from build123d import *

# Parameters (mm, degrees)
SKETCH_1_W               = 115
SKETCH_1_H               = 30
EXTRUDE_1_DEPTH          = 29
SHELL_1_T                = -2
SKETCH_4_W               = 55
SKETCH_4_H               = 63
EXTRUDE_2_DEPTH          = 2
SKETCH_7_W               = 28
SKETCH_7_H               = 49
CUT_EXTRUDE_2_DEPTH      = 28
EXTRUDE_6_DEPTH          = 29
EXTRUDE_8_DEPTH          = 2
EXTRUDE_9_DEPTH          = 115
FILLET_1_R               = 1
SKETCH_8_R               = 1.2
CUT_EXTRUDE_5_DEPTH      = 10
SKETCH_15_W              = 113
SKETCH_15_H              = 39.979543783
CUT_EXTRUDE_6_DEPTH      = 33
CUT_EXTRUDE_7_REACH      = 152.193
SKETCH_16_W              = 16.4
SKETCH_16_H              = 9.3
SKETCH_17_W              = 40.5
SKETCH_17_H              = 2
EXTRUDE_10_DEPTH         = 113
CUT_EXTRUDE_8_DEPTH      = 147
CUT_EXTRUDE_9_DEPTH      = 147
CUT_EXTRUDE_9_DEPTH_BACK = 147
SKETCH_21_W              = 20.17617045
SKETCH_21_H              = 57.30071962
SKETCH_22_W              = 2
SKETCH_22_H              = 5
CUT_EXTRUDE_11_DEPTH     = 0.2
SKETCH_24_W              = 113
SKETCH_24_H              = 56
EXTRUDE_16_DEPTH         = 0.2
CUT_EXTRUDE_12_DEPTH     = 147
CUT_EXTRUDE_13_DEPTH     = 5
FILLET_8_R               = 1
EXTRUDE_17_DEPTH         = 3
EXTRUDE_17_DEPTH_BACK    = 1
FILLET_10_R              = 1
SKETCH_28_W              = 115
SKETCH_28_H              = 5
EXTRUDE_18_DEPTH         = 1
CUT_EXTRUDE_START        = -3
CUT_EXTRUDE_14_DEPTH     = 3
CHAMFER_7_SIZE           = 3
FILLET_11_R              = 1


with BuildPart() as part:
    # Эскиз1 → Бобышка-Вытянуть1 (new body)
    with BuildSketch(Plane(origin=(0, 0, 0), x_dir=(1, 0, 0), z_dir=(0, 1, 0))):
        with Locations((57.5, 15)):
            Rectangle(SKETCH_1_W, SKETCH_1_H)
    extrude(amount=EXTRUDE_1_DEPTH)

    # Оболочка1
    shell_1_openings = [part.faces().sort_by_distance(p)[0] for p in [
        (57.5, 14.5, 0),
    ]]
    offset(amount=SHELL_1_T, openings=shell_1_openings, kind=Kind.INTERSECTION)

    # Эскиз4 → Бобышка-Вытянуть2 (add)
    with BuildSketch(Plane(origin=(115, 0, 0), x_dir=(0, 0, -1), z_dir=(1, 0, 0))):
        with Locations((15, 31.5)):
            Rectangle(SKETCH_4_W, SKETCH_4_H)
    extrude(amount=EXTRUDE_2_DEPTH)

    # Эскиз7 → Вырез-Вытянуть2 (cut)
    with BuildSketch(Plane(origin=(117, 0, 0), x_dir=(0, 0, -1), z_dir=(1, 0, 0))):
        with Locations((14, 31.5)):
            Rectangle(SKETCH_7_W, SKETCH_7_H)
    extrude(amount=-CUT_EXTRUDE_2_DEPTH, mode=Mode.SUBTRACT)

    # Эскиз10 → Бобышка-Вытянуть6 (add)
    with BuildSketch(Plane(origin=(0, 29, 0), x_dir=(1, 0, 0), z_dir=(0, 1, 0))):
        Polygon((115, 30), (115, 28), (89, 28), (2, 28), (2, 0), (0, 0), (0, 28), (0, 30), (87, 30), align=None)
    extrude(amount=EXTRUDE_6_DEPTH)

    # Эскиз13 → Бобышка-Вытянуть8 (add)
    with BuildSketch(Plane.XZ):
        Polygon((115, 12.5), (115, 40), (0, 40), (0, 0), (115, 0), align=None)
        with BuildLine():
            ThreePointArc((34.6, 31.75), (36.7, 33.85), (34.6, 35.95))
            Line((34.6, 35.95), (30.4, 35.95))
            ThreePointArc((30.4, 35.95), (28.3, 33.85), (30.4, 31.75))
            Line((30.4, 31.75), (34.6, 31.75))
        make_face(mode=Mode.SUBTRACT)
        with BuildLine():
            ThreePointArc((80.4, 35.95), (78.3, 33.85), (80.4, 31.75))
            Line((80.4, 31.75), (84.6, 31.75))
            ThreePointArc((84.6, 31.75), (86.7, 33.85), (84.6, 35.95))
            Line((84.6, 35.95), (80.4, 35.95))
        make_face(mode=Mode.SUBTRACT)
    extrude(amount=-EXTRUDE_8_DEPTH)

    # Эскиз14 → Бобышка-Вытянуть9 (add)
    with BuildSketch(Plane.ZY):
        with BuildLine():
            Line((-33.254799468, 26.65), (-33.254799468, 24.75))
            ThreePointArc((-33.254799468, 24.75), (-33.360427883, 24.57366508), (-33.565739508, 24.583589941))
            Line((-33.565739508, 24.583589941), (-36.254799468, 26.376296582))
            Line((-36.254799468, 26.376296582), (-36.254799468, 32.326296582))
            Line((-36.254799468, 32.326296582), (-33.565739508, 34.119003222))
            ThreePointArc((-33.565739508, 34.119003222), (-33.446213245, 34.269819382), (-33.254799468, 34.25))
            Line((-33.254799468, 34.25), (-33.254799468, 32.35))
            Line((-33.254799468, 32.35), (-30, 32.35))
            Line((-30, 32.35), (-30, 26.65))
            Line((-30, 26.65), (-33.254799468, 26.65))
        make_face()
        with BuildLine():
            Line((-33.254741117, 6.5), (-33.302994959, 4.600612844))
            ThreePointArc((-33.302994959, 4.600612844), (-33.462823881, 4.6084601), (-33.565739508, 4.730996778))
            Line((-33.565739508, 4.730996778), (-36.254799468, 6.523703418))
            Line((-36.254799468, 6.523703418), (-36.254799468, 12.473703418))
            Line((-36.254799468, 12.473703418), (-33.565739508, 14.266410059))
            ThreePointArc((-33.565739508, 14.266410059), (-33.360427883, 14.27633492), (-33.254799468, 14.1))
            Line((-33.254799468, 14.1), (-33.254799468, 12.2))
            Line((-33.254799468, 12.2), (-30, 12.2))
            Line((-30, 12.2), (-30, 6.5))
            Line((-30, 6.5), (-33.254741117, 6.5))
        make_face()
    extrude(amount=-EXTRUDE_9_DEPTH)

    # Скругление1
    fillet_1_edges = [part.edges().sort_by_distance(p)[0] for p in [
        (32.5, 0, 35.95),
        (82.5, 0, 35.95),
        (82.5, 0, 31.75),
        (78.3, 0, 33.85),
        (86.7, 0, 33.85),
        (36.7, 0, 33.85),
        (28.3, 0, 33.85),
        (32.5, 0, 31.75),
    ]]
    fillet(fillet_1_edges, radius=FILLET_1_R)

    # Эскиз8 → Вырез-Вытянуть5 (cut)
    with BuildSketch(Plane(origin=(117, 0, 0), x_dir=(0, 0, -1), z_dir=(1, 0, 0))):
        with Locations((-5.5, 31.5)):
            Circle(SKETCH_8_R)
    extrude(amount=-CUT_EXTRUDE_5_DEPTH, mode=Mode.SUBTRACT)

    # Эскиз15 → Вырез-Вытянуть6 (cut)
    with BuildSketch(Plane.XY.offset(-28)):
        with Locations((58.5, 46.989771892)):
            Rectangle(SKETCH_15_W, SKETCH_15_H)
    extrude(amount=CUT_EXTRUDE_6_DEPTH, mode=Mode.SUBTRACT)

    # Эскиз16 → Вырез-Вытянуть7 (cut, up to next)
    with BuildSketch(Plane(origin=(0, 0, -30), x_dir=(-1, 0, 0), z_dir=(0, 0, -1)), mode=Mode.PRIVATE) as cut_extrude_7_sk1:
        with Locations((-53.2, 49.65)):
            Rectangle(SKETCH_16_W, SKETCH_16_H)
    cut_extrude_7_tool1 = extrude(cut_extrude_7_sk1.sketch, amount=-CUT_EXTRUDE_7_REACH, mode=Mode.PRIVATE) & part.part
    add(cut_extrude_7_tool1.solids().sort_by_distance((53.2, 49.65, -30))[0], mode=Mode.SUBTRACT)

    # Эскиз17 → Бобышка-Вытянуть10 (add)
    with BuildSketch(Plane.ZY.offset(-115)):
        with Locations((-7.75, 57)):
            Rectangle(SKETCH_17_W, SKETCH_17_H)
    extrude(amount=EXTRUDE_10_DEPTH)

    # Эскиз20 → Вырез-Вытянуть8 (cut)
    with BuildSketch(Plane.ZY):
        Polygon((0, 2), (-27.8, 2), (-27.8, 71.965307459), (29.159484087, 71.965307459), (29.159484087, 2), align=None)
    extrude(amount=-CUT_EXTRUDE_8_DEPTH, mode=Mode.SUBTRACT)

    # Эскиз21 → Вырез-Вытянуть9 (cut, two sides: drawn at the far end of the back side and taken through both)
    with BuildSketch(Plane(origin=(0, 2, 0), x_dir=(1, 0, 0), z_dir=(0, 1, 0)).offset(-CUT_EXTRUDE_9_DEPTH_BACK)):
        with Locations((125.088085225, 16.15035981)):
            Rectangle(SKETCH_21_W, SKETCH_21_H)
    extrude(amount=CUT_EXTRUDE_9_DEPTH + CUT_EXTRUDE_9_DEPTH_BACK, mode=Mode.SUBTRACT)

    # Эскиз22 → Вырез-Вытянуть11 (cut)
    with BuildSketch(Plane.XY.offset(-28)):
        with Locations((114, 4.5)):
            Rectangle(SKETCH_22_W, SKETCH_22_H)
    extrude(amount=CUT_EXTRUDE_11_DEPTH, mode=Mode.SUBTRACT)

    # Эскиз24 → Бобышка-Вытянуть16 (add)
    with BuildSketch(Plane.XY.offset(-27.8)):
        with Locations((58.5, 28)):
            Rectangle(SKETCH_24_W, SKETCH_24_H)
    extrude(amount=-EXTRUDE_16_DEPTH)

    # Эскиз25 → Вырез-Вытянуть12 (cut)
    with BuildSketch(Plane(origin=(115, 0, 0), x_dir=(0, 0, -1), z_dir=(1, 0, 0))):
        Polygon((-61.35646419, 61.721146041), (45.258808631, 61.721146041), (45.258808631, 40.2), (-10.2, 40.2), (-10.2, -7.989940419), (-61.35646419, -7.989940419), (-61.35646419, 40.2), align=None)
    extrude(amount=-CUT_EXTRUDE_12_DEPTH, mode=Mode.SUBTRACT)

    # Эскиз26 → Вырез-Вытянуть13 (cut)
    with BuildSketch(Plane(origin=(0, 2, 0), x_dir=(1, 0, 0), z_dir=(0, 1, 0))):
        with BuildLine():
            Line((30.4, -2.1), (34.6, -2.1))
            ThreePointArc((34.6, -2.1), (36.7, -4.2), (34.6, -6.3))
            Line((34.6, -6.3), (30.4, -6.3))
            ThreePointArc((30.4, -6.3), (28.3, -4.2), (30.4, -2.1))
        make_face()
        with BuildLine():
            Line((80.4, -2.1), (84.6, -2.1))
            ThreePointArc((84.6, -2.1), (86.7, -4.2), (84.6, -6.3))
            Line((84.6, -6.3), (80.4, -6.3))
            ThreePointArc((80.4, -6.3), (78.3, -4.2), (80.4, -2.1))
        make_face()
    extrude(amount=-CUT_EXTRUDE_13_DEPTH, mode=Mode.SUBTRACT)

    # Скругление8
    fillet_8_edges = [part.edges().sort_by_distance(p)[0] for p in [
        (0, 3.25, -30),
        (0, 19.425, -30),
        (0, 36.275, -30),
        (0, 40.2, -28.9),
        (57.5, 40.2, -30),
        (115, 40.2, -28.9),
        (57.5, 0, 10.2),
        (57.5, 0, -30),
        (0, 0, -9.9),
    ]]
    fillet(fillet_8_edges, radius=FILLET_8_R)

    # Эскиз27 → Бобышка-Вытянуть17 (add, two sides: drawn at the far end of the back side and taken through both)
    with BuildSketch(Plane.XZ.offset(-EXTRUDE_17_DEPTH_BACK)):
        with BuildLine():
            Line((115, -30), (115, -29))
            Line((115, -29), (115, 9.2))
            Line((115, 9.2), (115, 10.2))
            Line((115, 10.2), (115, 15.2))
            Line((115, 15.2), (0, 15.2))
            Line((0, 15.2), (0, 10.2))
            Line((0, 10.2), (0, -29))
            ThreePointArc((0, -29), (0.292893219, -29.707106781), (1, -30))
            Line((1, -30), (115, -30))
        make_face()
        with BuildLine():
            Line((84.6, 6.3), (80.4, 6.3))
            ThreePointArc((80.4, 6.3), (78.3, 4.2), (80.4, 2.1))
            Line((80.4, 2.1), (84.6, 2.1))
            ThreePointArc((84.6, 2.1), (86.7, 4.2), (84.6, 6.3))
        make_face(mode=Mode.SUBTRACT)
        with BuildLine():
            Line((30.4, 2.1), (34.6, 2.1))
            ThreePointArc((34.6, 2.1), (36.7, 4.2), (34.6, 6.3))
            Line((34.6, 6.3), (30.4, 6.3))
            ThreePointArc((30.4, 6.3), (28.3, 4.2), (30.4, 2.1))
        make_face(mode=Mode.SUBTRACT)
    extrude(amount=EXTRUDE_17_DEPTH + EXTRUDE_17_DEPTH_BACK)

    # Скругление10
    fillet_10_edges = [part.edges().sort_by_distance(p)[0] for p in [
        (58, -3, -30),
        (0, -3, -6.9),
        (0.292893219, -3, -29.707106781),
    ]]
    fillet(fillet_10_edges, radius=FILLET_10_R)

    # Эскиз28 → Бобышка-Вытянуть18 (add)
    with BuildSketch(Plane(origin=(0, 1, 0), x_dir=(1, 0, 0), z_dir=(0, 1, 0))):
        with Locations((57.5, -12.7)):
            Rectangle(SKETCH_28_W, SKETCH_28_H)
    extrude(amount=EXTRUDE_18_DEPTH)

    # Эскиз29 → Вырез-Вытянуть14 (cut)
    # profile 1 of 2: a face of its own
    with BuildSketch(Plane.XZ.offset(3).offset(CUT_EXTRUDE_START)):
        with BuildLine():
            Line((30.4, 9.3), (34.6, 9.3))
            ThreePointArc((34.6, 9.3), (39.7, 4.2), (34.6, -0.9))
            Line((34.6, -0.9), (30.4, -0.9))
            ThreePointArc((30.4, -0.9), (25.3, 4.2), (30.4, 9.3))
        make_face()
        with BuildLine():
            Line((30.4, 2.1), (34.6, 2.1))
            ThreePointArc((34.6, 2.1), (36.7, 4.2), (34.6, 6.3))
            Line((34.6, 6.3), (30.4, 6.3))
            ThreePointArc((30.4, 6.3), (28.3, 4.2), (30.4, 2.1))
        make_face(mode=Mode.SUBTRACT)
    # profile 2 of 2: a face of its own
    with BuildSketch(Plane.XZ.offset(3).offset(CUT_EXTRUDE_START)):
        with BuildLine():
            Line((80.4, -0.9), (84.6, -0.9))
            ThreePointArc((84.6, -0.9), (89.7, 4.2), (84.6, 9.3))
            Line((84.6, 9.3), (80.4, 9.3))
            ThreePointArc((80.4, 9.3), (75.3, 4.2), (80.4, -0.9))
        make_face()
        with BuildLine():
            Line((80.4, 2.1), (84.6, 2.1))
            ThreePointArc((84.6, 2.1), (86.7, 4.2), (84.6, 6.3))
            Line((84.6, 6.3), (80.4, 6.3))
            ThreePointArc((80.4, 6.3), (78.3, 4.2), (80.4, 2.1))
        make_face(mode=Mode.SUBTRACT)
    extrude(amount=CUT_EXTRUDE_14_DEPTH, mode=Mode.SUBTRACT)

    # Фаска7
    chamfer_7_edges = [part.edges().sort_by_distance(p)[0] for p in [
        (82.5, -3, -0.9),
        (89.7, -3, 4.2),
        (75.3, -3, 4.2),
        (82.5, -3, 9.3),
        (32.5, -3, -0.9),
        (39.7, -3, 4.2),
        (25.3, -3, 4.2),
        (32.5, -3, 9.3),
    ]]
    chamfer(chamfer_7_edges, length=CHAMFER_7_SIZE - 0.0001)  # a hair under: the kernel refuses the full size

    # Скругление11
    fillet_11_edges = [part.edges().sort_by_distance(p)[0] for p in [
        (32.5, 0, 6.3),
        (28.3, 0, 4.2),
        (32.5, 0, 2.1),
        (36.7, 0, 4.2),
        (82.5, 0, 6.3),
        (78.3, 0, 4.2),
        (82.5, 0, 2.1),
        (86.7, 0, 4.2),
    ]]
    fillet(fillet_11_edges, radius=FILLET_11_R)


solid = part.part
The listing builds one solid part. Answer for the finished solid, in the listing's coordinates (mm). A direction names the side the tool comes from. Round coordinates to 2 decimals unless told otherwise and drop trailing zeros. Write each loop counter-clockwise with the first axis right and the second up, starting at its lowest first coordinate (ties: lowest second). Pieces come first, ordered by that corner, then holes. Notation, with made-up numbers: (61, -22) - (89, -22) arc R11 cw to (89, -4) - close; hole circle Ø6 at (-29.75, 46). An arc over 180 degrees is marked (long way). Use one line per item in the form item = value. Start each with the question number.
Item 1: Find the intervals of material crossed by line 1 (Z direction, x = 83.5, y = 36); line 2 (Z direction, x = 106, y = 27); line 3 (Y direction, x = 50, z = -2.5), in increasing order. Write a range as [from, to].
Item 2: A cutting plane is placed at D-D (z = -19). Write down the section's boundary in (x, y).
Item 3: A cutting plane is placed at B-B (x = 64). Write down the section's boundary in (y, z).
Item 4: Flat-ended cylindrical pins translate along their axes: pin 1 Ø5 at (x, z) = (80, 5) entering from -Y; pin 2 Ø1.5 at (x, y) = (17.5, 36) entering from +Z; pin 3 Ø1.5 at (x, z) = (18.5, -2.5) entering from +Y. Find the tip coordinate at first contact, or state that the pin passes through.
Item 5: A tool of negligible diameter and unlimited length cuts with its end or side. For faces 1 (the flat face through (57, 36, -30)), 2 (the flat face through (32.5, -1.5, -2.4)), 3 (the cylindrical face through (78.3, 1.5, 4.2)), 4 (the flat face through (56.695, 13.358, -34.929)), from which of +Z, -Z, +X, -X, +Y, -Y can it reach the whole face along a straight path? Write none if from no direction.
Item 6: A cutting plane is placed at A-A (z = 4.2). Give the number of separate pieces and of enclosed holes in the cut face, plus the area to 3 significant figures.
Item 7: A cutting plane is placed at C-C (y = 20). Write down the section's boundary in (x, z), plus the area to 3 significant figures.
Item 8: Determine the mould class of faces 5 (the flat face through (56.695, 5.615, -34.891)), 6 (the flat face through (57, 26.65, -32)), 7 (the cylindrical face through (86.7, 1.5, 4.2)) for opening direction Y: +Y half, -Y half, draft (parallel to the pull), parting line (faces both ways), or undercut.
The answers:
q1.line_1 = [-30, -27.8]
q1.line_2 = [-36.25, -27.8]
q1.line_3 = [-3, 2]
q2.outline = (0, -2) arc R1 ccw to (1, -3) - (115, -3) - (115, 2) - (0, 2) - close
q3.outline = (-3, -29) arc R1 ccw to (-2, -30) - (6.5, -30) - (6.5, -33.25) - (4.6, -33.3) arc R0.2 ccw to (4.73, -33.57) - (6.52, -36.25) - (12.47, -36.25) - (14.27, -33.57) arc R0.2 ccw to (14.1, -33.25) - (12.2, -33.25) - (12.2, -30) - (26.65, -30) - (26.65, -33.25) - (24.75, -33.25) arc R0.2 ccw to (24.58, -33.57) - (26.38, -36.25) - (32.33, -36.25) - (34.12, -33.57) arc R0.2 ccw to (34.25, -33.25) - (32.35, -33.25) - (32.35, -30) - (39.2, -30) arc R1 ccw to (40.2, -29) - (40.2, -27.8) - (2, -27.8) - (2, 15.2) - (-3, 15.2) - close
q4.pin_1 = 0
q4.pin_2 = -27.8
q4.pin_3 = 2
q5.face_1 = +X, -X, +Y
q5.face_2 = -Y
q5.face_3 = +Y, -Y
q5.face_4 = -Z, +X, -X
q6.separate_pieces = 3
q6.enclosed_holes = 0
q6.area = 436 mm^2
q7.outline = (0, -29) arc R1 ccw to (1, -30) - (115, -30) - (115, -27.8) - (0, -27.8) - close
q7.area = 253 mm^2
q8.face_5 = -Y half
q8.face_6 = undercut
q8.face_7 = draft
